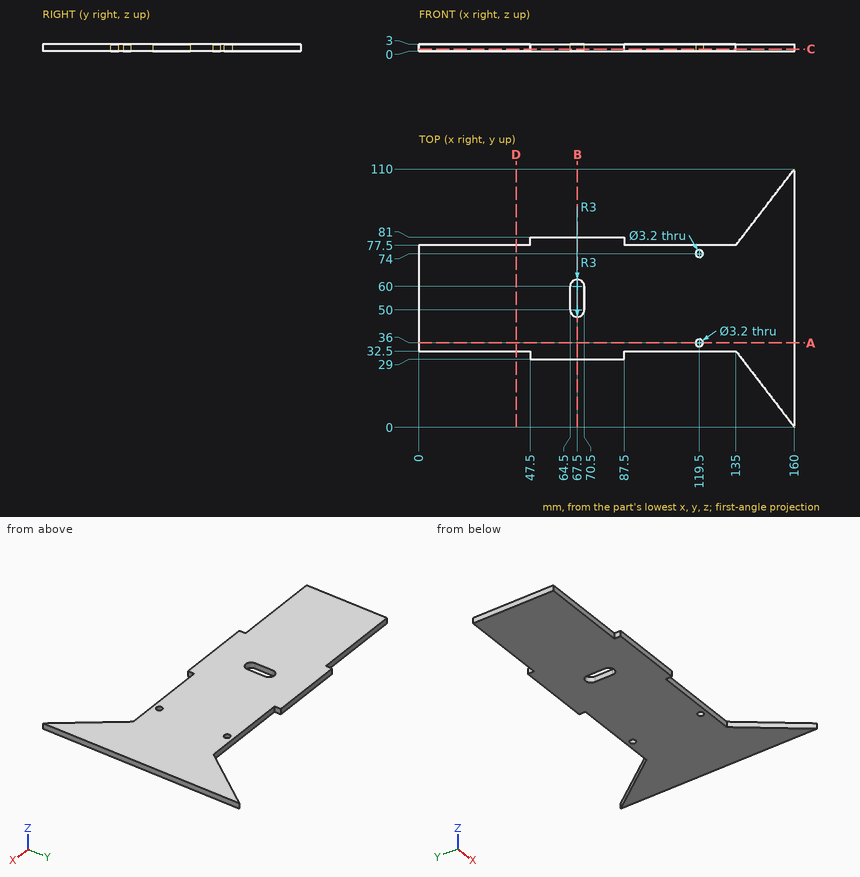
Answer from the drawing. Dimensions are ordinates in mm from the lowest x, y and z of the part. Give positions to 0.01 mm unless a question says otherwise; leave off trailing zeros. Loops run counter-clockwise (first coordinate to the right, second up) from the corner with the lowest first, then second, coordinate; pieces in that order, holes last. Notation, with made-up numbers: (54, -14) - (59, -14) arc R24 ccw to (59, 8) - close; hole circle Ø4 at (-37.75, 2.5). An arc over 180 degrees is marked (long way). Answer as a JSON object with one key per item and string values.
1. Flat-ended cylindrical pins translate along their axes: pin 1 Ø4 at (x, y) = (119.5, 74) entering from +Z; pin 2 Ø1.5 at (x, z) = (32, 0.5) entering from -Y; pin 3 Ø1.5 at (x, z) = (19.5, 1.5) entering from +Y; pin 4 Ø1.5 at (y, z) = (80, 2) entering from -X. Find the tip coordinate at first contact, or state that the pin passes through.
Determined:
{"pin 1": "z = 3", "pin 2": "y = 32.5", "pin 3": "y = 77.5", "pin 4": "x = 47.5"}
2. A cutting plane is placed at C-C (z = 0.85). Write down the section's boundary in (x, y), then the cut area to 3 significant figures.
Determined:
{"outline": "(0, 32.5) - (47.5, 32.5) - (47.5, 29) - (87.5, 29) - (87.5, 32.5) - (135, 32.5) - (160, 0) - (160, 110) - (135, 77.5) - (87.5, 77.5) - (87.5, 81) - (47.5, 81) - (47.5, 77.5) - (0, 77.5) - close; hole (64.5, 50) arc R3 ccw to (70.5, 50) - (70.5, 60) arc R3 ccw to (64.5, 60) - close; hole circle Ø3.2 at (119.5, 36); hole circle Ø3.2 at (119.5, 74)", "area": "8,190 mm²"}
3. A cutting plane is placed at B-B (x = 67.5). Write down the section's boundary in (y, z).
Determined:
{"outline": "(29, 0) - (47, 0) - (47, 3) - (29, 3) - close; (63, 0) - (81, 0) - (81, 3) - (63, 3) - close"}
4. A cutting plane is placed at D-D (x = 41.5). Write down the section's boundary in (y, z).
Determined:
{"outline": "(32.5, 0) - (77.5, 0) - (77.5, 3) - (32.5, 3) - close"}
5. A cutting plane is placed at A-A (y = 36). Write down the section's boundary in (x, z).
Determined:
{"outline": "(0, 0) - (117.9, 0) - (117.9, 3) - (0, 3) - close; (121.1, 0) - (160, 0) - (160, 3) - (121.1, 3) - close"}
6. Find the intervals of material crossed by L1, parallel to Y at x = 119.5, z = 0.95; L2, parallel to X at y = 74, z = 1.9; L3, parallel to X at y = 56, z = 2.5, in increasing order. Write a range as [from, to].
Determined:
{"L1": "[32.5, 34.4], [37.6, 72.4], [75.6, 77.5]", "L2": "[0, 117.9], [121.1, 160]", "L3": "[0, 64.5], [70.5, 160]"}
